Source: CAD feature listing. Evaluate the final solid. Frame: model axes, mm. A direction names the side the tool comes from. Round coordinates to 2 decimals unless told otherwise and drop trailing zeros. Write each loop counter-clockwise with the first axis right and the second up, starting at its lowest first coordinate (ties: lowest second). Pieces come first, ordered by that corner, then holes.
from build123d import *

# Parameters (mm, degrees)
BOSS_EXTRUDE1_DEPTH = 7
SKETCH2_R           = 1.45
CUT_EXTRUDE1_DEPTH  = 7.5
SKETCH3_R           = 1.45
CUT_EXTRUDE2_DEPTH  = 7.5


with BuildPart() as part:
    # Sketch1 → Boss-Extrude1 (new body)
    with BuildSketch(Plane(origin=(0, 0, 0), x_dir=(0, 0, -1), z_dir=(1, 0, 0))):
        Polygon((0, 0), (0, 10.2), (9, 10.2), (15.9, 21.2), (24.3, 21.2), (24.3, 0), align=None)
    extrude(amount=BOSS_EXTRUDE1_DEPTH)

    # Sketch2 → Cut-Extrude1 (cut)
    with BuildSketch(Plane.XZ):
        with Locations((3.5, -5.35)):
            Circle(SKETCH2_R)
        with Locations((3.5, -14.75)):
            Circle(SKETCH2_R)
    extrude(amount=-CUT_EXTRUDE1_DEPTH, mode=Mode.SUBTRACT)

    # Sketch3 → Cut-Extrude2 (cut)
    with BuildSketch(Plane(origin=(0, 0, -24.3), x_dir=(-1, 0, 0), z_dir=(0, 0, -1))):
        with Locations((-3.5, 15.75)):
            Circle(SKETCH3_R)
        with Locations((-3.5, 5.35)):
            Circle(SKETCH3_R)
    extrude(amount=-CUT_EXTRUDE2_DEPTH, mode=Mode.SUBTRACT)


solid = part.part
1) Section query A-A on x = 3.5. Return the cut outline in (y, z).
Taken from the geometry:
outline: (0, -24.3) - (3.9, -24.3) - (3.9, -16.8) - (6.8, -16.8) - (6.8, -24.3) - (14.3, -24.3) - (14.3, -16.8) - (17.2, -16.8) - (17.2, -24.3) - (21.2, -24.3) - (21.2, -15.9) - (10.2, -9) - (10.2, 0) - (0, 0) - (0, -3.9) - (7.5, -3.9) - (7.5, -6.8) - (0, -6.8) - (0, -13.3) - (7.5, -13.3) - (7.5, -16.2) - (0, -16.2) - close
2) Section query C-C on y = 1.75. Return the cut outline in (x, z).
Taken from the geometry:
outline: (0, -24.3) - (7, -24.3) - (7, 0) - (0, 0) - close; hole circle Ø2.9 at (3.5, -14.75); hole circle Ø2.9 at (3.5, -5.35)
3) Section query D-D on z = -18.75. Return the cut outline in (x, y).
Taken from the geometry:
outline: (0, 0) - (7, 0) - (7, 21.2) - (0, 21.2) - close; hole circle Ø2.9 at (3.5, 5.35); hole circle Ø2.9 at (3.5, 15.75)
4) Material intervals for line 1 (Y direction, x = 3.5, z = -18.25); line 2 (Z direction, x = 3.5, y = 3.75); line 3 (Z direction, x = 3.5, y = 5), sorted ascending.
Taken from the geometry:
line 1: y = 0 to 3.9, 6.8 to 14.3, 17.2 to 21.2
line 2: z = -24.3 to -16.2, -13.3 to -6.8, -3.9 to 0
line 3: z = -16.8 to -16.2, -13.3 to -6.8, -3.9 to 0
5) Reachability of faces 1 (the face through (4, 16, -16.8)), 2 (the face through (3, 10.2, -4)), 3 (the face through (3, 21.2, -20)), 4 (the face through (3, 7.5, -15)) from +Z, -Z, +X, -X, +Y, -Y: full face, straight path, thin tool, end or side. Return the list, or none.
Taken from the geometry:
face 1: -Z
face 2: +Z, +X, -X, +Y
face 3: +Z, -Z, +X, -X, +Y
face 4: -Y
6) Contact query for flat-ended pins moving along their axis: P1, Ø0.9, axis at x = 4, y = 16, coming from the -Z side; P2, Ø1.4, axis at x = 3.5, z = -14.5, coming from the -Y side; P3, Ø3.5, axis at x = 3.5, y = 15.75, coming from the +Z side. Output: stop coordinate, or through.
Taken from the geometry:
P1: stops at z = -16.8
P2: stops at y = 7.5
P3: stops at z = -11.38
7) Section query B-B on z = -5.35. Return the cut outline in (x, y), then the cut area to 4 significant figures.
Taken from the geometry:
outline: (0, 0) - (2.05, 0) - (2.05, 7.5) - (4.95, 7.5) - (4.95, 0) - (7, 0) - (7, 10.2) - (0, 10.2) - close
area: 49.65 mm2
8) Pull-direction query (X, two-part tool) for faces 5 (the face through (7, 8, -15)), 6 (the face through (3, 11, -24.3)), 7 (the face through (4.65, 4.47, -20.6)); classes: released by +X, released by -X, zero draft, split by the parting line, or undercut.
Taken from the geometry:
face 5: released by +X
face 6: zero draft
face 7: undercut
